from build123d import *

# Parameters (mm, degrees)
SKETCH4_R           = 43.057541212
BOSS_EXTRUDE1_DEPTH = 41.5


with BuildPart() as part:
    # Sketch3 → Revolve1 (revolve)
    with BuildSketch(Plane(origin=(0, 0, 0), x_dir=(0, 0, -1), z_dir=(1, 0, 0))):
        Polygon((0, 0), (217, 0), (217, 24.8), (182, 24.8), (182, 27.500000118), (169.1, 27.500000118), (169.1, 36), (160.1, 36), (160.1, 30), (18.1, 30), (18.1, 32.5), (11.1, 32.5), (11.1, 25), (0, 25), align=None)
    revolve(axis=Axis((0, 0, 0), (0, 0, -1)))

    # Sketch4 → Boss-Extrude1 (add, symmetric)
    with BuildSketch(Plane.XY.offset(-105.1)):
        Circle(SKETCH4_R)
    extrude(amount=BOSS_EXTRUDE1_DEPTH, both=True)


solid = part.part
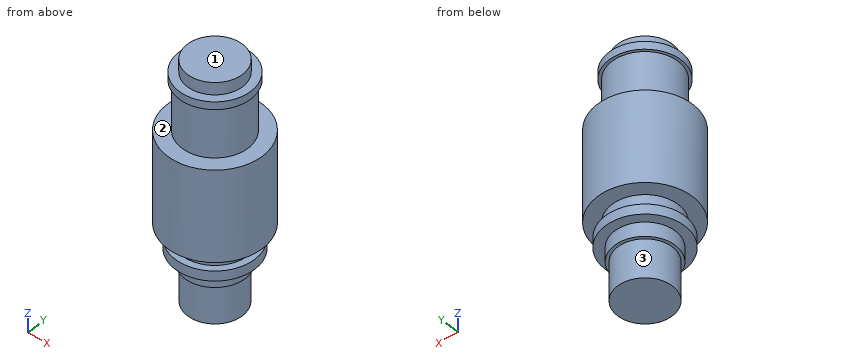
The model under review builds one solid part; all positions refer to its coordinate system, in mm. Face numbers are marked on the shaded views. A direction names the side the tool comes from. Give positions to 0.01 mm unless a question says otherwise; leave off trailing zeros. Order: outer loops, then holes, each group sorted by start corner. A loop starts at its lowest first (then second) coordinate and runs counter-clockwise, first axis right, second up. Notation, with made-up numbers: M -18.5,-22 L 28.5,-22 A18 ccw 28.5,8 Z; hole C 89,52.5 d3. An arc over 180 degrees is marked long. One line per question, with ' | ' between items. Start each with the question number.
1) Clearance check with flat-ended pins moving along their axes: P1, Ø1.5, axis at x = -24.5, y = -21, coming from the +Z side; P2, Ø6, axis at x = -11.5, z = -143, coming from the +Y side; P3, Ø4, axis at y = -4, z = -170, coming from the +X side. State where each tip first meets the part, or that it passes through.
2) Consider section D-D, the plane z = -122. Give the boundary of the cut face in (x, y).
3) Consider section C-C, the plane z = -59. Give the boundary of the cut face in (x, y), then the cut area to 3 significant figures.
4) For the marked faces 1, 2 and 3, list the 3-axis set-ups (+Z, -Z, +X, -X, +Y, -Y) from which the entire face can be reached by the end or side of a thin tool; tool diameter is ignored.
5) Wall thickness on L1, parallel to Z at x = -30, y = -4.5; L2, parallel to X at y = -1, z = -139; L3, parallel to Y at x = 2, z = -106.5: over which ranges is each line inside the solid? List them lowest first. Write a range as from..to.
Found:
1) P1: stops at z = -11.1 | P2: stops at y = 42.21 | P3: stops at x = 35.93
2) outline: C 0,0 d86.12
3) outline: C 0,0 d60 | area: 2,830 mm²
4) face 1: +Z, +X, -X, +Y, -Y | face 2: none | face 3: -Z
5) L1: z = -169.1..-160.1, -146.6..-63.6, -18.1..-11.1 | L2: x = -43.05..43.05 | L3: y = -43.01..43.01
